Design review of the part built by this model. Coordinates are the model's own, in mm. A direction names the side the tool comes from. Round coordinates to 2 decimals unless told otherwise and drop trailing zeros. Order: outer loops, then holes, each group sorted by start corner. A loop starts at its lowest first (then second) coordinate and runs counter-clockwise, first axis right, second up. Notation, with made-up numbers: (-18, 38.5) - (36, 38.5) arc R25 cw to (36, 51.5) - close; hole circle Ø1 at (6.25, 73). An arc over 180 degrees is marked (long way). Use CSV: the item, a comma, the result in double quotes.
Autodesk Inventor part; units mm, degrees
ref_plane "Work Plane1" through (-120, 0, 0) normal (1, 0, 0) x (0, 1, 0)
ref_plane "XZ Plane" through (0, 0, 0) normal (0, 1, 0) x (-1, 0, 0)
ref_plane "XY Plane" through (0, 0, 0) normal (0, 0, 1) x (1, 0, 0)
sketch "Sketch1" plane through (0, 0, 0) normal (0, 1, 0) x (-1, 0, 0)
  line L0 (0, 0) -> (40, 0)
  line L1 (90, 50) -> (90, 150)
  arc A0 (40, 0) -> (90, 50) centre (40, 50) ccw
  point P0 (90, 0)
  dimension "d0" = 90
  dimension "d1" = 150
  dimension "d2" = 50
sketch "Sketch2" plane through (0, 0, 0) normal (1, 0, 0) x (0, 1, 0)
  circle A0 centre (0, 0) radius 25
  dimension "d3" = 50
sweep "Sweep1" add profiles "Sketch2" path "Sketch1"
shell "Shell1" thickness 5 removed faces 2 at (0, -6.2376, 1.5374) at (-91.9943, -6.0822, 150)
sketch "Sketch3" plane through (0, 0, 0) normal (1, 0, 0) x (0, 0, -1)
  circle A0 centre (0, 0) radius 26
  circle A1 centre (0, 0) radius 25
  dimension "d7" = 52
extrude "Extrusion1" add sketch "Sketch3" against normal blind 20
sketch "Sketch5" plane through (-90, 0, 150) normal (0, 0, 1) x (1, 0, 0)
  circle A0 centre (0, 0) radius 24.13
  circle A1 centre (0, 0) radius 25
  point P0 (90, 0)
  dimension "d11" = 48.26
extrude "Extrusion2" cut sketch "Sketch5" against normal blind 50
ref_plane "Work Plane1" through (-120, 0, 0) normal (1, 0, 0) x (0, 1, 0)
sketch "Sketch6" plane through (-120, 0, 0) normal (1, 0, 0) x (0, 1, 0)
  circle A0 centre (0, 0) radius 6
  dimension "d15" = 12
extrude "Extrusion3" add sketch "Sketch6" along normal up to surface
sketch "Sketch8" plane through (-120, 0, 0) normal (-1, 0, 0) x (0, 0, 1)
  circle A0 centre (0, 0) radius 3.5
  dimension "d22" = 7
extrude "Extrusion4" cut sketch "Sketch8" against normal through all
sketch "Sketch9" plane through (0, 0, 0) normal (1, 0, 0) x (0, 0, -1)
  circle A0 centre (0, 0) radius 22.5
  circle A1 centre (0, 0) radius 20
  dimension "d25" = 45
extrude "Extrusion5" cut sketch "Sketch9" against normal blind 15
properties part number "FEE-PIPE"
1) We need section C-C (y = 0). Give the number of separate pieces and of enclosed holes in the cut face, then the cut area to 3 significant figures.
Data:
separate pieces,"3"
enclosed holes,"0"
area,"2,140 mm2"
2) Insertion check: pin 1 Ø2 at (x, y) = (-99, -13.5) entering from -Z; pin 2 Ø8 at (x, z) = (-61.5, 40.5) entering from -Y; pin 3 Ø6 at (x, z) = (-60, 8.5) entering from -Y; pin 4 Ø4 at (y, z) = (0, 0) entering from -X. Each pin has a flat end and moves straight along its axis. Give the tip position at first contact, or say it passes through.
Data:
pin 1,"stops at z = 8.61"
pin 2,"stops at y = -10.91"
pin 3,"stops at y = -24.98"
pin 4,"passes through"
3) For faces 1 (the face through (-103.1, 20.5, 100)), 2 (the face through (-15, -1.6, 20.1)), 3 (the face through (-20, 21, 14)), list the 3-axis set-ups (+Z, -Z, +X, -X, +Y, -Y) from which the entire face can be reached by the end or side of a thin tool; tool diameter is ignored.
Data:
face 1,"+Z"
face 2,"+X"
face 3,"none"
4) To check wall thickness, follow L1, parallel to Y at x = -98, z = 0; L2, parallel to Y at x = -5.5, z = 0; L3, parallel to Z at x = -34, y = 0. State the ranges of each line that lie inside material, in increasing order. Write a range as from..to.
Data:
L1,"y = -6..-3.5, 3.5..6"
L2,"y = -26..-22.5, 22.5..26"
L3,"z = -25..-20, 20..25"
5) We need section A-A (y = -13). Give the boundary of the cut face in (x, z).
Data:
outline,"(-111.35, 50) arc R71.35 ccw to (-40, -21.35) - (-20, -21.35) - (-20, -22.52) - (0, -22.52) - (0, -18.36) - (-15, -18.36) - (-15, -15.2) - (-40, -15.2) arc R65.2 cw to (-105.2, 50) - (-105.2, 150) - (-110.33, 150) - (-110.33, 100) - (-111.35, 100) - close; (-74.8, 50) arc R34.8 ccw to (-40, 15.2) - (-15, 15.2) - (-15, 18.36) - (0, 18.36) - (0, 22.52) - (-20, 22.52) - (-20, 21.35) - (-40, 21.35) arc R28.65 cw to (-68.65, 50) - (-68.65, 100) - (-69.67, 100) - (-69.67, 150) - (-74.8, 150) - close"
6) We need section B-B (z = 93). Give the boundary of the cut face in (x, y).
Data:
outline,"circle Ø50 at (-90, 0); hole circle Ø40 at (-90, 0)"
7) The part is to be moulded in two halves that separate along Z. For faces 4 (the face through (-9.86, -15.821, 20.633)), 5 (the face through (0, 19.4, 11.7)), 6 (the face through (-108.5, -0.78, -5.95)), 7 (the face through (-93, 20, 150)), say which applies: +Z half, -Z half, draft (parallel to the pull), parting line (faces both ways), or undercut.
Data:
face 4,"parting line"
face 5,"draft"
face 6,"undercut"
face 7,"+Z half"
